Build history of the part. All positions in model axes, mm. Round coordinates to 2 decimals unless told otherwise and drop trailing zeros. Order: outer loops, then holes, each group sorted by start corner. A loop starts at its lowest first (then second) coordinate and runs counter-clockwise, first axis right, second up. Notation, with made-up numbers: (57, 41) -> (104, 41) arc R34 ccw to (104, 71) -> close; hole circle Ø9 at (88.25, -35). An arc over 180 degrees is marked (long way). Answer as CSV lines item,"result". Start each with the question number.
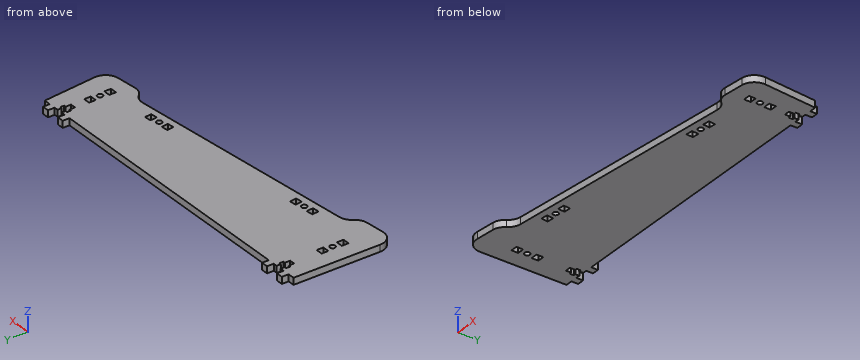
```python
from build123d import *

# Parameters (mm, degrees)
ESQUISSE1_W        = 5
ESQUISSE1_H        = 5
ESQUISSE1_R        = 2
BOSS_EXTRU_1_DEPTH = 5
CONG_1_R           = 10


with BuildPart() as part:
    # Esquisse1 → Boss.-Extru.1 (new body)
    with BuildSketch(Plane.XY):
        Polygon((15, 0), (10, 0), (10, 5), (5, 5), (5, 0), (2, 0), (2, -3), (3.5, -3), (3.5, -6), (2, -6), (2, -10), (-2, -10), (-2, -6), (-3.5, -6), (-3.5, -3), (-2, -3), (-2, 0), (-5, 0), (-5, 5), (-10, 5), (-10, 0), (-15, 0), (-15, -75.371818049), (14.852006469, -72.395627572), (20.02875697, -63.839854419), (205.344258903, -45.364237629), (212.108310991, -52.729534592), (241.96031746, -49.753344116), (237, 0), (232, 0), (232, 5), (227, 5), (227, 0), (224, 0), (224, -3), (225.5, -3), (225.5, -6), (224, -6), (224, -10), (220, -10), (220, -6), (218.5, -6), (218.5, -3), (220, -3), (220, 0), (217, 0), (217, 5), (212, 5), (212, 0), (207, 0), align=None)
        with Locations((0, -47.5)):
            Rectangle(ESQUISSE1_W, ESQUISSE1_H, mode=Mode.SUBTRACT)
        Polygon((42.039762682, -51.595821645), (42.535794429, -56.571156057), (37.560460017, -57.067187803), (37.064428271, -52.091853391), align=None, mode=Mode.SUBTRACT)
        with Locations((47.263112967, -53.587457105)):
            Circle(ESQUISSE1_R, mode=Mode.SUBTRACT)
        with Locations((0, -40)):
            Circle(ESQUISSE1_R, mode=Mode.SUBTRACT)
        Polygon((57.461797663, -55.083060818), (52.486463252, -55.579092564), (51.990431506, -50.603758153), (56.965765917, -50.107726407), align=None, mode=Mode.SUBTRACT)
        Polygon((171.398457383, -38.698996248), (171.894489129, -43.67433066), (166.919154718, -44.170362406), (166.423122972, -39.195027994), align=None, mode=Mode.SUBTRACT)
        with Locations((176.621807668, -40.690631708)):
            Circle(ESQUISSE1_R, mode=Mode.SUBTRACT)
        Polygon((186.820492364, -42.186235422), (181.845157952, -42.682267168), (181.349126206, -37.706932756), (186.324460618, -37.21090101), align=None, mode=Mode.SUBTRACT)
        with Locations((222, -37.5)):
            Rectangle(ESQUISSE1_W, ESQUISSE1_H, mode=Mode.SUBTRACT)
        with Locations((0, -32.5)):
            Rectangle(ESQUISSE1_W, ESQUISSE1_H, mode=Mode.SUBTRACT)
        with Locations((222, -30)):
            Circle(ESQUISSE1_R, mode=Mode.SUBTRACT)
        with Locations((222, -22.5)):
            Rectangle(ESQUISSE1_W, ESQUISSE1_H, mode=Mode.SUBTRACT)
    extrude(amount=BOSS_EXTRU_1_DEPTH)

    # Congé1
    cong_1_edges = [part.edges().sort_by_distance(p)[0] for p in [
        (241.96031746, -49.753344116, 2.5),
        (205.344258903, -45.364237629, 2.5),
        (212.108310991, -52.729534592, 2.5),
        (-15, -75.371818049, 2.5),
        (20.02875697, -63.839854419, 2.5),
        (14.852006469, -72.395627572, 2.5),
    ]]
    fillet(cong_1_edges, radius=CONG_1_R - 0.0001)  # a hair under: the kernel refuses the full size


solid = part.part
```
Q1. Slice it at B-B, the plane x = 101.5. Write the cut outline in (y, z).
Q2. Flat gauge pins, fed straight in: pin 1 Ø1.5 at (x, z) = (1, 2) entering from +Y; pin 2 Ø1.5 at (y, z) = (-4.5, 3.5) entering from +X; pin 3 Ø2.5 at (y, z) = (-5, 1.5) entering from +X. Where does each tip first touch, or does it go through?
Q3. Slice it at A-A, the plane z = 3.45. Count the separate pieces of the cut face and the enclosed holes in it, plus the area to 3 significant figures.
Q4. Probe L1, parallel to X at y = -0.5, z = 1; L2, parallel to Y at x = 0, z = 2.35; L3, parallel to X at y = -7, z = 1. List the from-to ranges inside material, lowest first.
Q5. Slice it at C-C, the plane x = 14. Write the cut outline in (y, z).
Solutions:
1,outline,"(-55.72, 0) -> (0, 0) -> (0, 5) -> (-55.72, 5) -> close"
2,pin 1,"stops at y = -10"
2,pin 2,"stops at x = 237.52"
2,pin 3,"stops at x = 237.62"
3,separate pieces,"1"
3,enclosed holes,"12"
3,area,"14,100 mm2"
4,L1,"x = -15 to -2, 2 to 220, 224 to 237.05"
4,L2,"y = -73.88 to -50, -45 to -42, -38 to -35, -30 to -10"
4,L3,"x = -15 to -2, 2 to 220, 224 to 237.7"
5,outline,"(-71.53, 0) -> (0, 0) -> (0, 5) -> (-71.53, 5) -> close"
